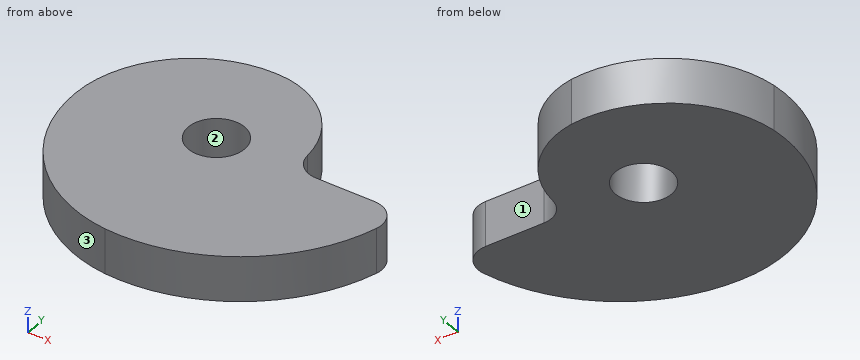
from build123d import *

# Parameters (mm, degrees)
SKETCH1_R           = 3
BOSS_EXTRUDE1_DEPTH = 2.4
FILLET1_R           = 2.6


with BuildPart() as part:
    # Sketch1 → Boss-Extrude1 (new body, symmetric)
    with BuildSketch(Plane.XY):
        with BuildLine():
            Line((8, 0), (20, 0))
            ThreePointArc((20, 0), (13.52081528, -12.642135624), (0, -17))
            ThreePointArc((0, -17), (-10.52081528, -11.399494937), (-14, 0))
            ThreePointArc((-14, 0), (-9.278174593, 8.399494937), (0, 11))
            ThreePointArc((0, 11), (6.278174593, 7.156854249), (8, 0))
        make_face()
        Circle(SKETCH1_R, mode=Mode.SUBTRACT)
    extrude(amount=BOSS_EXTRUDE1_DEPTH, both=True)

    # Fillet1
    fillet1_edges = [part.edges().sort_by_distance(p)[0] for p in [
        (8, 0, 0),
        (20, 0, 0),
    ]]
    fillet(fillet1_edges, radius=FILLET1_R)


solid = part.part
Build history of the part. All positions in model axes, mm. Face numbers are marked on the shaded views. Give positions to 0.01 mm unless a question says otherwise; leave off trailing zeros. Write each loop counter-clockwise with the first axis right and the second up, starting at its lowest first coordinate (ties: lowest second). Pieces come first, ordered by that corner, then holes. Notation, with made-up numbers: (32, -2.5) - (45, -2.5) arc R11 ccw to (45, 8.5) - close; hole circle Ø8 at (71.5, 20). An arc over 180 degrees is marked (long way). Use one line per item in the form item = value. Start each with the question number.
1. Two-plate mould, pull along X, no slides. Class the marked faces 1, 2 and 3: released by +X, released by -X, zero draft, split by the parting line, or undercut.
2. Band-saw the part on A-A on z = 1.7. Write the cut outline in (x, y).
3. Band-saw the part on C-C on y = -13.5. Write the cut outline in (x, z), plus the area to 3 significant figures.
4. Band-saw the part on B-B on x = -10. Write the cut outline in (y, z), plus the area to 3 significant figures.
5. Probe line 1 (Y direction, x = 0, z = -1.3); line 2 (X direction, y = 2, z = 0.4); line 3 (X direction, y = 1.5, z = 1.2). List the from-to ranges inside material, lowest first. Write a range as [from, to].
6. Drop flat-ended pins along their axis: pin 1 Ø2.5 at (x, z) = (14, -0.5) entering from +Y; pin 2 Ø2 at (y, z) = (-12.5, 2) entering from +X; pin 3 Ø2 at (y, z) = (-8.5, 0.5) entering from -X. Give the stop position or say it passes through.
Conclusion:
q1.face_1 = zero draft
q1.face_2 = undercut
q1.face_3 = released by -X
q2.outline = (-14, 0) arc R15.57 ccw to (0, -17) arc R18.56 ccw to (19.44, -3.27) arc R2.6 ccw to (16.93, 0) - (10.67, 0) arc R2.6 cw to (8.08, 2.37) arc R9.62 ccw to (0, 11) arc R12.59 ccw to start; hole circle Ø6 at (0, 0)
q3.outline = (-8.42, -2.4) - (12.43, -2.4) - (12.43, 2.4) - (-8.42, 2.4) - close
q3.area = 100 mm²
q4.outline = (-12, -2.4) - (7.79, -2.4) - (7.79, 2.4) - (-12, 2.4) - close
q4.area = 95.0 mm²
q5.line_1 = [-17, -3], [3, 11]
q5.line_2 = [-13.59, -2.24], [2.24, 8.14]
q5.line_3 = [-13.73, -2.6], [2.6, 8.31]
q6.pin_1 = 0
q6.pin_2 = 14.75
q6.pin_3 = -12.87
